from build123d import *

# Parameters (mm, degrees)
PROFILE_EXTRUDE_DEPTH         = 31.75
INTERIOR_START                = -3
INTERIOR_SKETCH_W             = 57.5
INTERIOR_SKETCH_H             = 37.4
INTERIOR_CUT_DEPTH            = 50
OPENING_CUT_REACH             = 77.925
OPENING_SKETCH_W              = 47.5
OPENING_SKETCH_H              = 27.4
INSIDE_TOP_CHAMFER_SIZE       = 5
INSIDE_FILLETS_R              = 1
WIRE_OUTLET_CUT_REACH         = 77.925
WIRE_OUTLET_CUT_SKETCH_R      = 9.5
WIRE_OUTLET_FILLET_R          = 1.5
TOP_FILLETS_R                 = 4
M4_MOUNTING_SCREWS_AT_2_COUNT = 2
M4_MOUNTING_SCREWS_AT_2_PITCH = 35.5


with BuildPart() as part:
    # Profile Sketch → Profile Extrude (new, symmetric)
    with BuildSketch(Plane(origin=(0, 0, 0), x_dir=(0, 0, -1), z_dir=(1, 0, 0))):
        Polygon((0, 0), (0, 43.6), (-20, 43.6), (-20, 53.6), (43.4, 53.6), (43.4, 0), align=None)
    extrude(amount=PROFILE_EXTRUDE_DEPTH, both=True)

    # Interior Sketch → Interior Cut (cut)
    with BuildSketch(Plane.XZ.offset(INTERIOR_START)):
        with Locations((0, -21.7)):
            Rectangle(INTERIOR_SKETCH_W, INTERIOR_SKETCH_H)
    extrude(amount=-INTERIOR_CUT_DEPTH, mode=Mode.SUBTRACT)

    # Opening Sketch → Opening Cut (cut, up to next)
    with BuildSketch(Plane(origin=(0, 53.6, 0), x_dir=(1, 0, 0), z_dir=(0, 1, 0)), mode=Mode.PRIVATE) as opening_cut_sk1:
        with Locations((0, 21.7)):
            Rectangle(OPENING_SKETCH_W, OPENING_SKETCH_H)
    opening_cut_tool1 = extrude(opening_cut_sk1.sketch, amount=-OPENING_CUT_REACH, mode=Mode.PRIVATE) & part.part
    add(opening_cut_tool1.solids().sort_by_distance((0, 53.6, -21.7))[0], mode=Mode.SUBTRACT)

    # Inside Top Chamfer
    inside_top_chamfer_edges = [part.edges().sort_by_distance(p)[0] for p in [
        (0, 53, -3),
        (28.75, 53, -21.7),
        (0, 53, -40.4),
        (-28.75, 53, -21.7),
    ]]
    chamfer(inside_top_chamfer_edges, length=INSIDE_TOP_CHAMFER_SIZE - 0.0001)  # a hair under: the kernel refuses the full size

    # Inside Fillets
    inside_fillets_edges = [part.edges().sort_by_distance(p)[0] for p in [
        (28.75, 25.50005, -40.4),
        (28.75, 25.50005, -3),
        (-28.75, 25.50005, -40.4),
        (-28.75, 25.50005, -3),
    ]]
    fillet(inside_fillets_edges, radius=INSIDE_FILLETS_R)

    # Wire Outlet Cut Sketch → Wire Outlet Cut (cut, up to next)
    with BuildSketch(Plane.XZ, mode=Mode.PRIVATE) as wire_outlet_cut_sk1:
        with Locations(Location((0, -21.7, 0), (0, 0, 270))):
            Circle(WIRE_OUTLET_CUT_SKETCH_R)
    wire_outlet_cut_tool1 = extrude(wire_outlet_cut_sk1.sketch, amount=-WIRE_OUTLET_CUT_REACH, mode=Mode.PRIVATE) & part.part
    add(wire_outlet_cut_tool1.solids().sort_by_distance((0, 0, -21.7))[0], mode=Mode.SUBTRACT)

    # Wire Outlet Fillet
    wire_outlet_fillet_edges = [part.edges().sort_by_distance(p)[0] for p in [
        (0, 0, -12.2),
        (0, 3, -12.2),
    ]]
    fillet(wire_outlet_fillet_edges, radius=WIRE_OUTLET_FILLET_R - 0.0001)  # a hair under: the kernel refuses the full size

    # Top Fillets
    top_fillets_edges = [part.edges().sort_by_distance(p)[0] for p in [
        (0, 0, 0),
        (0, 53.6, 20),
        (0, 53.6, -43.4),
        (0, 0, -43.4),
        (31.75, 53.6, -11.7),
        (31.75, 48.6, 20),
        (31.75, 21.8, 0),
        (31.75, 0, -21.7),
        (-31.75, 21.8, 0),
        (-31.75, 48.6, 20),
        (-31.75, 53.6, -11.7),
        (-31.75, 26.8, -43.4),
        (-31.75, 0, -21.7),
        (31.75, 26.8, -43.4),
    ]]
    fillet(top_fillets_edges, radius=TOP_FILLETS_R)

    # M4 Mounting Screws Profile Sketch → M4 Mounting Screws (revolve, cut)
    with BuildSketch(Plane(origin=(-17.75, 53.6, 10), x_dir=(0, 0, 1), z_dir=(1, 0, 0))):
        Polygon((0, 0), (0, 10), (2.25, 10), (2.25, 3.45), (4.7, 1), (4.7, 0), align=None)
    m4_mounting_screws = revolve(axis=Axis((-17.75, 59.95, 10), (0, -1, 0)), mode=Mode.SUBTRACT)

    # M4 Mounting Screws at 2: M4 Mounting Screws ×2
    with Locations(*[(i * M4_MOUNTING_SCREWS_AT_2_PITCH, 0, 0) for i in range(1, M4_MOUNTING_SCREWS_AT_2_COUNT)]):
        add(m4_mounting_screws, mode=Mode.SUBTRACT)


solid = part.part
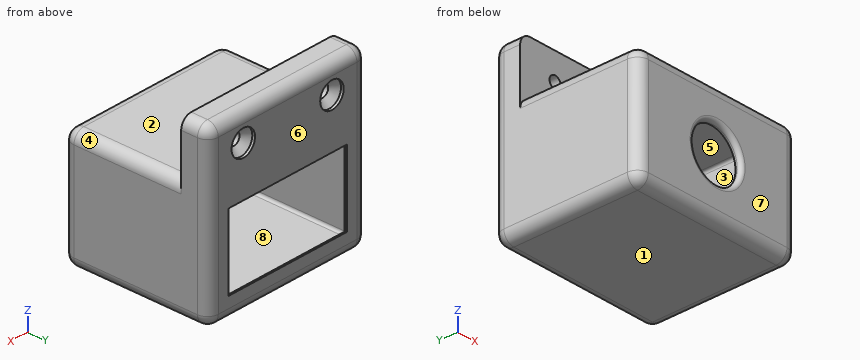
CAD build for the part. Positions are in the model's coordinates, mm. Face numbers are marked on the shaded views. A direction names the side the tool comes from. Round coordinates to 2 decimals unless told otherwise and drop trailing zeros. Loops run counter-clockwise (first coordinate to the right, second up) from the corner with the lowest first, then second, coordinate; pieces in that order, holes last. Notation, with made-up numbers: M 3.5,89.5 L 60.5,89.5 A22 ccw 60.5,112.5 Z; hole C -2,5.25 d9. An arc over 180 degrees is marked long. One line per question, with ' | ' between items. Start each with the question number.
Item 1: Two-plate mould, pull along Y, no slides. Class the marked faces 5, 6, 7 and 8: pulls with the +Y half, pulls with the -Y half, needs draft (parallel to the pull), parting line crosses it, or undercut.
Item 2: Wall check: line 1 (X direction, y = 47, z = 10); line 2 (Z direction, x = -17.75, y = 45.75); line 3 (Z direction, x = -27, y = 15). Give the ranges that are in metal, low to high.
Item 3: Cut at A-A, the plane z = 10. Write the cut outline in (x, y).
Item 4: Cut at D-D, the plane y = 24. Write the cut outline in (x, z).
Item 5: Pin check, flat tips, straight feed: pin 1 Ø19 at (x, z) = (-7.5, 8.5) entering from -Y; pin 2 Ø0.7 at (y, z) = (53.5, -22.5) entering from +X; pin 3 Ø22 at (x, z) = (0, -21.7) entering from +Y. Stop position of each tip, or through.
Item 6: Which spindle directions (+Z, -Z, +X, -X, +Y, -Y) get a long thin tool onto all of the face, cutting with end or side? Do the marked faces 1, 2, 3 and 4. Say none if no direction does.
Responses:
1) face 5: undercut | face 6: pulls with the +Y half | face 7: pulls with the -Y half | face 8: undercut
2) line 1: x = -31.75 to -20, -15.5 to 15.5, 20 to 31.75 | line 2: z = -43.4 to -40.4, -3 to 7.75, 12.25 to 20 | line 3: z = -43.4 to -40.4, -3 to 0
3) outline: M -31.75,43.6 L -20,43.6 L -20,50.15 L -22.45,52.6 L -22.45,53.6 L -27.75,53.6 A4 ccw -31.75,49.6 Z; M -15.5,43.6 L 15.5,43.6 L 15.5,50.15 L 13.05,52.6 L 13.05,53.6 L -13.05,53.6 L -13.05,52.6 L -15.5,50.15 Z; M 20,43.6 L 31.75,43.6 L 31.75,49.6 A4 ccw 27.75,53.6 L 22.45,53.6 L 22.45,52.6 L 20,50.15 Z
4) outline: M -31.75,-39.4 A4 ccw -27.75,-43.4 L 27.75,-43.4 A4 ccw 31.75,-39.4 L 31.75,-4 A4 ccw 27.75,0 L -27.75,0 A4 ccw -31.75,-4 Z; hole M -28.75,-39.4 A1 ccw -27.75,-40.4 L 27.75,-40.4 A1 ccw 28.75,-39.4 L 28.75,-4 A1 ccw 27.75,-3 L -27.75,-3 A1 ccw -28.75,-4 Z
5) pin 1: stops at y = 1.35 | pin 2: stops at x = 29.59 | pin 3: stops at y = 3
6) face 1: -Z, +X, -X, +Y, -Y | face 2: +Z, +X, -X, -Y | face 3: none | face 4: +Z, +X, -Y
